```python
from build123d import *

# Parameters (mm, degrees)
BOSS_EXTRUDE1_DEPTH = 12.9
FILLET1_R           = 5
FILLET2_R           = 1
FILLET3_R           = 0.5


with BuildPart() as part:
    # Sketch2 → Boss-Extrude1 (new body)
    with BuildSketch(Plane(origin=(-7.378322523, 7.378322523, 0), x_dir=(0, 0, 1), z_dir=(-0.7071067811865452, 0.7071067811865498, 0))):
        with BuildLine():
            Line((56.29999994, -16.741883092), (56.29999994, -19.091883092))
            Line((56.29999994, -19.091883092), (16.29999994, -19.091883092))
            Line((16.29999994, -19.091883092), (16.29999994, -16.741883092))
            Line((16.29999994, -16.741883092), (18.421835943, -16.741883092))
            ThreePointArc((18.421835943, -16.741883092), (21.641004351, -17.201790003), (22.591287788, -14.091883092))
            Line((22.591287788, -14.091883092), (22.29999994, -14.091883092))
            Line((22.29999994, -14.091883092), (21.612440415, -14.091883092))
            ThreePointArc((21.612440415, -14.091883092), (21.863334003, -14.564164788), (21.94999994, -15.091883092))
            ThreePointArc((21.94999994, -15.091883092), (18.821402632, -15.824174018), (21.29999994, -13.779442617))
            Line((21.29999994, -13.779442617), (21.29999994, -13.091883092))
            Line((21.29999994, -13.091883092), (21.29999994, -12.800595245))
            ThreePointArc((21.29999994, -12.800595245), (19.756303769, -12.651720296), (18.421835943, -13.441883092))
            Line((18.421835943, -13.441883092), (16.29999994, -13.441883092))
            Line((16.29999994, -13.441883092), (16.29999994, 15.258116908))
            Line((16.29999994, 15.258116908), (18.421835943, 15.258116908))
            ThreePointArc((18.421835943, 15.258116908), (19.756303769, 14.467954112), (21.29999994, 14.61682906))
            Line((21.29999994, 14.61682906), (21.29999994, 14.908116908))
            Line((21.29999994, 14.908116908), (21.29999994, 15.595676433))
            ThreePointArc((21.29999994, 15.595676433), (18.821402632, 17.640407834), (21.94999994, 16.908116908))
            ThreePointArc((21.94999994, 16.908116908), (21.863334003, 16.380398604), (21.612440415, 15.908116908))
            Line((21.612440415, 15.908116908), (22.29999994, 15.908116908))
            Line((22.29999994, 15.908116908), (22.591287788, 15.908116908))
            ThreePointArc((22.591287788, 15.908116908), (21.641004351, 19.018023818), (18.421835943, 18.558116908))
            Line((18.421835943, 18.558116908), (16.29999994, 18.558116908))
            Line((16.29999994, 18.558116908), (16.29999994, 22.908116908))
            Line((16.29999994, 22.908116908), (14.29999994, 22.908116908))
            Line((14.29999994, 22.908116908), (14.29999994, -21.091883092))
            Line((14.29999994, -21.091883092), (58.29999994, -21.091883092))
            Line((58.29999994, -21.091883092), (58.29999994, 22.908116908))
            Line((58.29999994, 22.908116908), (56.29999994, 22.908116908))
            Line((56.29999994, 22.908116908), (56.29999994, 18.558116541))
            Line((56.29999994, 18.558116541), (54.178163937, 18.558116908))
            ThreePointArc((54.178163937, 18.558116908), (50.95899553, 19.018023818), (50.008712093, 15.908116908))
            Line((50.008712093, 15.908116908), (50.29999994, 15.908116908))
            Line((50.29999994, 15.908116908), (50.987559466, 15.908116908))
            ThreePointArc((50.987559466, 15.908116908), (51.772281637, 18.471450971), (53.94999994, 16.908116908))
            ThreePointArc((53.94999994, 16.908116908), (53.032290866, 15.4295196), (51.29999994, 15.595676433))
            Line((51.29999994, 15.595676433), (51.29999994, 14.908116908))
            Line((51.29999994, 14.908116908), (51.29999994, 14.61682906))
            ThreePointArc((51.29999994, 14.61682906), (52.843696112, 14.467954112), (54.178163937, 15.258116908))
            Line((54.178163937, 15.258116908), (56.29999994, 15.258116908))
            Line((56.29999994, 15.258116908), (56.29999994, -13.441883092))
            Line((56.29999994, -13.441883092), (54.178163937, -13.441883092))
            ThreePointArc((54.178163937, -13.441883092), (52.843696112, -12.651720296), (51.29999994, -12.800595245))
            Line((51.29999994, -12.800595245), (51.29999994, -13.091883092))
            Line((51.29999994, -13.091883092), (51.29999994, -13.779442617))
            ThreePointArc((51.29999994, -13.779442617), (53.032290866, -13.613285784), (53.94999994, -15.091883092))
            ThreePointArc((53.94999994, -15.091883092), (51.772281637, -16.655217155), (50.987559466, -14.091883092))
            Line((50.987559466, -14.091883092), (50.29999994, -14.091883092))
            Line((50.29999994, -14.091883092), (50.008712093, -14.091883092))
            ThreePointArc((50.008712093, -14.091883092), (50.95899553, -17.201790003), (54.178163937, -16.741883092))
            Line((54.178163937, -16.741883092), (56.29999994, -16.741883092))
        make_face()
    extrude(amount=BOSS_EXTRUDE1_DEPTH)

    # Fillet1
    # the kernel refuses this fillet: 5 mm, written as the material it adds along each edge
    with BuildSketch(Plane(origin=(-20.878322523, -6.121677477, 56.29999994), x_dir=(0, 0, -1), z_dir=(-0.7071067811865452, 0.7071067811865498, 0))) as fillet1_piece_1:
        with BuildLine():
            CenterArc((4.239988208, -5), FILLET1_R, 90, 57.994545172)
            Line((0, -2.35), (-0.084799764, -2.297))
            ThreePointArc((-0.084799764, -2.297), (-0.1, -1.175), (-0.1, 0))
            Line((-0.1, 0), (0, 0.1))
            Line((0, 0.1), (4.239988208, 0.1))
            Line((4.239988208, 0.1), (4.239988208, 0))
        make_face()
    extrude(amount=12.9)
    with BuildSketch(Plane(origin=(-20.878322523, -6.121677477, 16.29999994), x_dir=(0.7071067811865498, 0.7071067811865452, 4.67144053935759e-13), z_dir=(-0.7071067811865452, 0.7071067811865498, 0))) as fillet1_piece_2:
        with BuildLine():
            CenterArc((5, -4.239988208), FILLET1_R, 122.005454828, 57.994545172)
            Line((0, -4.239988208), (-0.1, -4.239988208))
            Line((-0.1, -4.239988208), (-0.1, 0))
            Line((-0.1, 0), (0, 0.1))
            ThreePointArc((0, 0.1), (1.175, 0.1), (2.297, 0.084799764))
            Line((2.297, 0.084799764), (2.35, 0))
        make_face()
    extrude(amount=12.9)

    # Fillet2
    # the kernel refuses this fillet: 1 mm, written as the material it adds along each edge
    with BuildSketch(Plane(origin=(-19.216621587, -4.459976542, 16.29999994), x_dir=(-0.4742981469837023, -0.4742981469836992, 0.7416754920689071), z_dir=(-0.7071067811865452, 0.7071067811865498, 0))) as fillet2_piece_1:
        with BuildLine():
            CenterArc((2.460931793, 0.961889952), FILLET2_R, 152.5257211, 133.343162112)
            Line((1.573713762, 1.423240324), (1.555969401, 1.432467331))
            ThreePointArc((1.555969401, 1.432467331), (0.773441703, 0.726453672), (-0.013415177, 0.01483351))
            Line((-0.013415177, 0.01483351), (-0.005468737, -0.019237799))
            ThreePointArc((-0.005468737, -0.019237799), (1.367184329, -0.210550238), (2.739837396, -0.019237799))
            Line((2.739837396, -0.019237799), (2.734368658, 0))
        make_face()
    extrude(amount=12.9)
    with BuildSketch(Plane(origin=(-19.216621587, -4.459976542, 56.29999994), x_dir=(-0.47429814698388373, -0.4742981469838806, -0.7416754920686752), z_dir=(-0.7071067811865452, 0.7071067811865498, 0))) as fillet2_piece_2:
        with BuildLine():
            CenterArc((2.460931793, -0.961889952), FILLET2_R, 74.131116788, 133.343162112)
            Line((1.573713762, -1.423240324), (1.555969401, -1.432467331))
            ThreePointArc((1.555969401, -1.432467331), (0.773441703, -0.726453672), (-0.013415177, -0.01483351))
            Line((-0.013415177, -0.01483351), (-0.005468737, 0.019237799))
            ThreePointArc((-0.005468737, 0.019237799), (1.367184329, 0.210550238), (2.739837396, 0.019237799))
            Line((2.739837396, 0.019237799), (2.734368658, 0))
        make_face()
    extrude(amount=12.9)

    # Fillet3
    fillet3_edges = [part.edges().sort_by_distance(p)[0] for p in [
        (-23.777460326, 0.100862197, 18.421835943),
        (-23.777460326, 0.100862197, 54.178163937),
    ]]
    fillet(fillet3_edges, radius=FILLET3_R)


solid = part.part
```
Can you work these out from the model? Positions are in its coordinate system, mm. A direction names the side the tool comes from. Round coordinates to 2 decimals unless told otherwise and drop trailing zeros. Loops run counter-clockwise (first coordinate to the right, second up) from the corner with the lowest first, then second, coordinate; pieces in that order, holes last. Notation, with made-up numbers: M 87,13 L 122,13 A10 ccw 122,24 Z; hole C 20.25,29 d2. An arc over 180 degrees is marked long. Answer as a JSON object with one key per item and string values. Group by question number.
Q1. Will these pins go through, and if not, where does the flat tip stop? pin 1 (2 mm diameter, centred on y = 26.5, z = 47.5, fed in from -X); pin 2 (12 mm diameter, centred on y = -2.5, z = 27.5, fed in from +X); pin 3 (2 mm diameter, centred on y = -2.5, z = 29, fed in from -X); pin 4 (6 mm diameter, centred on x = -22, z = 29, fed in from +Y).
Q2. We'd pull the mould along Z, two halves only. Please class faces 1 (the flat face through (-11, 12, 58.3)), 2 (the flat face through (-1.2, 22.6, 51.3)), 3 (the flat face through (-21.766, -7.009, 33.603)): +Z half, -Z half, draft (parallel to the pull), parting line (faces both ways), or undercut.
Q3. Please list where these lines run through material, in increasing order: L1, parallel to Z at x = 3.5, y = 24.5; L2, parallel to Z at x = -2.5, y = 25.5; L3, parallel to Z at x = -18, y = -0.5.
Q4. Imagine slicing it at B-B, the plane x = -7. Please give me the cut outline in (y, z).
Q5. On a 3-axis mill with a long thin cutter (end or side, diameter ignored), from which of +Z, -Z, +X, -X, +Y, -Y can I reach the whole of each face in a straight line? I mean faces 4 (the flat face through (-11, 13, 14.3)), 5 (the flat face through (-0.6, 23.1, 22.1)), 6 (the flat face through (-11, 12, 16.3)), 7 (the flat face through (1.247, 24.998, 55.254)). Say none if no direction works.
Q6. Imagine slicing it at C-C, the plane z = 37.5. Please give me the cut outline in (x, y).
Q7. Imagine slicing it at A-A, the plane y = 9.5. Please give me the cut outline in (x, z).
Findings:
{
 "1": {"pin 1": "passes through", "pin 2": "stops at x = -17.34", "pin 3": "stops at x = -28.33", "pin 4": "stops at y = -2"},
 "2": {"face 1": "+Z half", "face 2": "undercut", "face 3": "draft"},
 "3": {"L1": "z = 14.3 to 16.3, 56.3 to 58.3", "L2": "z = 14.3 to 18.78, 21.82 to 22.72, 49.88 to 50.78, 53.82 to 58.3", "L3": "z = 14.3 to 16.3, 18.81 to 21.3, 51.3 to 53.79, 56.3 to 58.3"},
 "4": {"outline": "M 7.76,14.3 L 26,14.3 L 26,16.3 L 7.76,16.3 Z; M 7.76,56.3 L 26,56.3 L 26,58.3 L 7.76,58.3 Z"},
 "5": {"face 4": "-Z, +X, -X, +Y, -Y", "face 5": "-X, -Y", "face 6": "none", "face 7": "+X, +Y"},
 "6": {"outline": "M -31.41,1.59 L -22.29,-7.54 L -20.88,-6.12 L -30,3 Z"},
 "7": {"outline": "M -23.5,14.3 L -5.26,14.3 L -5.26,16.3 L -23.5,16.3 Z; M -23.5,56.3 L -5.26,56.3 L -5.26,58.3 L -23.5,58.3 Z"}
}
